Verification items for this drawing (mm, ordinates from the low corner). A direction names the side the tool comes from. Give positions to 0.01 mm unless a question says otherwise; leave off trailing zeros. Loops run counter-clockwise (first coordinate to the right, second up) from the corner with the lowest first, then second, coordinate; pieces in that order, holes last. Notation, with made-up numbers: (28.5, 5) -> (80.5, 5) arc R31 cw to (80.5, 36) -> close; hole circle Ø9 at (-34.5, -14). An arc over 180 degrees is marked (long way). Write each question's results on one line, items separated by ' | '. Start each with the question number.
Item 1: Scan lines: line 1 along Z through (x, y) = (29, 4.75); line 2 along Z through (x, y) = (27.5, 8.25); line 3 along Y through (x, z) = (16, 78). Record each from-to range of solid material in increasing order.
Item 2: Cross-section at A-A on x = 5. Enter the section's corners in (y, z), then the cut area to 3 significant figures.
Item 3: Access from +Z, -Z, +X, -X, +Y, -Y to the whole of each face (thin tool, end or side, straight path). Record for the marked faces 1, 2 and 3.
Item 4: Gauge pin test, flat ends, axial feed: pin 1 Ø1 at (y, z) = (2.5, 68) entering from +X; pin 2 Ø4 at (x, z) = (7, 37) entering from -Y; pin 3 Ø4 at (y, z) = (7.5, 33.5) entering from -X; pin 4 Ø1 at (y, z) = (6.5, 75) entering from -X. Record the tip position at first contact, or that the pin passes through.
Item 5: Cross-section at B-B on y = 5. Enter the section's corners in (x, z), then the cut area to 3 significant figures.
Item 6: Cross-section at C-C on y = 9. Enter the section's corners in (x, z), then the cut area to 3 significant figures.
Item 7: Cross-section at D-D on z = 25. Enter the section's corners in (x, y), then the cut area to 3 significant figures.
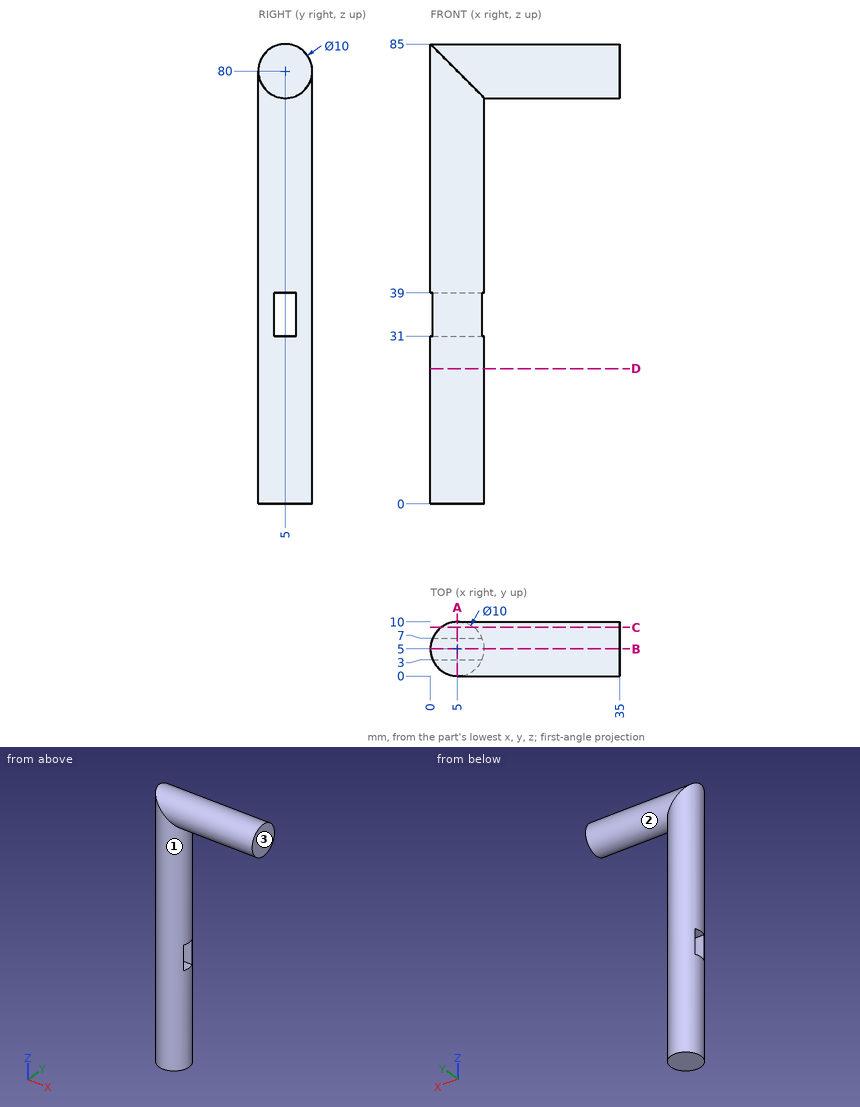
Answer sheet:
1) line 1: z = 75.01 to 84.99 | line 2: z = 76.2 to 83.8 | line 3: y = 0.42 to 9.58
2) outline: (0, 0) -> (10, 0) -> (10, 80) arc R5 ccw to (0, 80) -> close; hole (3, 31) -> (7, 31) -> (7, 39) -> (3, 39) -> close | area: 807 mm²
3) face 1: -Z | face 2: +X | face 3: +Z, -Z, +X, +Y, -Y
4) pin 1: stops at x = 9.58 | pin 2: stops at y = 0 | pin 3: stops at x = 0.42 | pin 4: stops at x = 0.1
5) outline: (0, 0) -> (10, 0) -> (10, 31) -> (0, 31) -> close; (0, 39) -> (10, 39) -> (10, 75) -> (35, 75) -> (35, 85) -> (0, 85) -> close | area: 1,020 mm²
6) outline: (2, 0) -> (8, 0) -> (8, 77) -> (35, 77) -> (35, 83) -> (2, 83) -> close | area: 660 mm²
7) outline: circle Ø10 at (5, 5) | area: 78.5 mm²
